```python
from build123d import *

# Parameters (mm, degrees)
SKETCH1_W           = 130
SKETCH1_H           = 145
SKETCH1_R           = 6.45
BOSS_EXTRUDE1_DEPTH = 15
CHAMFER1_SIZE       = 80
FILLET2_R           = 25
FILLET1_R           = 2
BOSS_EXTRUDE2_DEPTH = 130
SKETCH3_R           = 2.75
CUT_EXTRUDE1_DEPTH  = 45
SKETCH4_R           = 1.5
CUT_EXTRUDE2_DEPTH  = 25


with BuildPart() as part:
    # Sketch1 → Boss-Extrude1 (new body)
    with BuildSketch(Plane.XY):
        with Locations((65, 72.5)):
            Rectangle(SKETCH1_W, SKETCH1_H)
        with Locations((60, 60)):
            Circle(SKETCH1_R, mode=Mode.SUBTRACT)
        with Locations((106.669047558, 106.669047558)):
            Circle(SKETCH1_R, mode=Mode.SUBTRACT)
        with Locations((16.179114569, 34.7)):
            Circle(SKETCH1_R, mode=Mode.SUBTRACT)
    extrude(amount=BOSS_EXTRUDE1_DEPTH)

    # Chamfer1
    chamfer1_edges = [part.edges().sort_by_distance(p)[0] for p in [
        (0, 145, 7.5),
    ]]
    chamfer(chamfer1_edges, length=CHAMFER1_SIZE)

    # Fillet2
    fillet2_edges = [part.edges().sort_by_distance(p)[0] for p in [
        (0, 65, 7.5),
    ]]
    fillet(fillet2_edges, radius=FILLET2_R)

    # Fillet1
    fillet1_edges = [part.edges().sort_by_distance(p)[0] for p in [
        (80, 145, 7.5),
        (130, 145, 7.5),
    ]]
    fillet(fillet1_edges, radius=FILLET1_R)

    # Sketch2 → Boss-Extrude2 (add, through all)
    with BuildSketch(Plane(origin=(130, 0, 0), x_dir=(0, 0, -1), z_dir=(1, 0, 0))):
        Polygon((0, 15), (15, 0), (0, 0), align=None)
    extrude(amount=-BOSS_EXTRUDE2_DEPTH)

    # Sketch3 → Cut-Extrude1 (cut)
    with BuildSketch(Plane.XZ):
        with Locations((35, 7.5)):
            Circle(SKETCH3_R)
        with Locations((105, 7.5)):
            Circle(SKETCH3_R)
    extrude(amount=-CUT_EXTRUDE1_DEPTH, mode=Mode.SUBTRACT)

    # Sketch4 → Cut-Extrude2 (cut)
    with BuildSketch(Plane(origin=(0, 145, 0), x_dir=(1, 0, 0), z_dir=(0, 1, 0))):
        with Locations((121, -7.5)):
            Circle(SKETCH4_R)
        with Locations((88, -7.5)):
            Circle(SKETCH4_R)
    extrude(amount=-CUT_EXTRUDE2_DEPTH, mode=Mode.SUBTRACT)


solid = part.part
```
CAD build for the part. Positions are in the model's coordinates, mm. A direction names the side the tool comes from. Round coordinates to 2 decimals unless told otherwise and drop trailing zeros. Write each loop counter-clockwise with the first axis right and the second up, starting at its lowest first coordinate (ties: lowest second). Pieces come first, ordered by that corner, then holes. Notation, with made-up numbers: (53.5, -10) -> (89.5, -10) arc R23 cw to (89.5, 4) -> close; hole circle Ø4 at (-21.75, 31). An arc over 180 degrees is marked (long way). Answer in a Markdown table with one row per item. Add a question column.
Item 1: Which spindle directions (+Z, -Z, +X, -X, +Y, -Y) get a long thin tool onto all of the face, cutting with end or side? Do faces 1 (the face through (130, 73, 6)), 2 (the face through (79, 66, 0)), 3 (the face through (119.5, 132.68, 7.43)), 4 (the face through (35, 45, 8)). Say none if no direction does.
Item 2: Saw through at D-D, the plane y = 60. Write the cut outline in (x, z), then the cut area to 3 significant figures.
Item 3: Saw through at A-A, the plane y = 34.7. Write the cut outline in (x, z).
Item 4: Mould opens along X. For faces 5 (the face through (22.137, 32.23, 7.395)), 6 (the face through (0, 22, 6)), 7 (the face through (104, 145, 7)) say: pulls with the +X half, pulls with the -X half, needs draft (parallel to the pull), parting line crosses it, or undercut.
Item 5: Drill centre lines: line 1 (X direction, y = 132.75, z = 7.5); line 2 (Z direction, x = 124.5, y = 106); line 3 (X direction, y = 111, z = 4.5). Where is each one in solid material? Low to high. Write a range as from..to.
Item 6: Saw through at B-B, the plane x = 60. Write the cut outline in (y, z).
Item 7: Drop flat-ended pins along their axis: pin 1 Ø3 at (x, z) = (105, 9) entering from -Y; pin 2 Ø11.5 at (x, y) = (60, 60) entering from -Z; pin 3 Ø8 at (x, y) = (112, 71.5) entering from -Z; pin 4 Ø1.5 at (x, z) = (88.5, 7.5) entering from +Y. Give the stop position or say it passes through.
Item 8: Saw through at C-C, the plane x = 35. Write the cut outline in (y, z), then the cut area to 4 significant figures.
Findings below:
| question | item | result |
|---|---|---|
| 1 | face 1 | +Z, -Z, +X, +Y, -Y |
| 1 | face 2 | -Z, +X, -X, +Y |
| 1 | face 3 | +Y |
| 1 | face 4 | -Y |
| 2 | outline | (0.58, 0) -> (53.55, 0) -> (53.55, 15) -> (0.58, 15) -> close; (66.45, 0) -> (130, 0) -> (130, 15) -> (66.45, 15) -> close |
| 2 | area | 1,750 mm^2 |
| 3 | outline | (0, 0) -> (9.73, 0) -> (9.73, 15) -> (0, 15) -> close; (22.63, 0) -> (130, 0) -> (130, 15) -> (22.63, 15) -> close; hole circle Ø5.5 at (35, 7.5); hole circle Ø5.5 at (105, 7.5) |
| 4 | face 5 | undercut |
| 4 | face 6 | pulls with the -X half |
| 4 | face 7 | needs draft |
| 5 | line 1 | x = 67.75..86.5, 89.5..119.5, 122.5..130 |
| 5 | line 2 | z = 0..15 |
| 5 | line 3 | x = 46..101.89, 111.45..130 |
| 6 | outline | (0, -15) -> (15, 0) -> (53.55, 0) -> (53.55, 15) -> (0, 15) -> close; (66.45, 0) -> (125, 0) -> (125, 15) -> (66.45, 15) -> close |
| 7 | pin 1 | stops at y = 0 |
| 7 | pin 2 | passes through |
| 7 | pin 3 | stops at z = 0 |
| 7 | pin 4 | stops at y = 120 |
| 8 | outline | (0, -15) -> (15, 0) -> (100, 0) -> (100, 15) -> (0, 15) -> (0, 10.25) -> (45, 10.25) -> (45, 4.75) -> (0, 4.75) -> close |
| 8 | area | 1,365 mm^2 |
